The model under review builds one solid part; all positions refer to its coordinate system, in mm. A direction names the side the tool comes from. Coordinates: 2 decimals unless noted, no trailing zeros. Write each loop counter-clockwise with the first axis right and the second up, starting at its lowest first coordinate (ties: lowest second). Pieces come first, ordered by that corner, then holes. Notation, with made-up numbers: (34.25, 70.25) - (69.25, 70.25) arc R26 cw to (69.25, 90.25) - close; hole circle Ø5 at (-8.75, -38). An arc over 180 degrees is marked (long way). Put each result on its own line as item: value. Start each with the question number.
Item 1: Consider section C-C on z = 177.8. Give the boundary of the cut face in (x, y).
Item 2: Consider section B-B on x = 259. Give the boundary of the cut face in (y, z).
Item 3: Mouldability with a two-part tool opening along Z and no side actions: class faces 4 (the face through (-305, 188, -247.65)), 5 (the face through (5, 0, -4)), 6 (the face through (244, 127, 177)) as pulls with the +Z half, pulls with the -Z half, needs draft (parallel to the pull), parting line crosses it, or undercut.
Item 4: For pin 1 (5 mm diameter, centred on y = 232.5, z = -250, fed in from +X); pin 2 (15 mm diameter, centred on x = 11, y = 207, fed in from -Z), all flat-tipped, find the tip position at first contact; note any pin that passes through.
Item 5: To check wall thickness, follow L1, parallel to X at y = 75, z = -177; L2, parallel to X at y = 46.5, z = 177.8; L3, parallel to X at y = 342.5, z = -9. State the ranges of each line that lie inside material, in increasing order. Write a range as [from, to].
Item 6: Consider section D-D on x = 12.5. Give the boundary of the cut face in (y, z).
Item 7: Consider section A-A on z = 0. Give the boundary of the cut face in (x, y), then the cut area to 3 significant figures.
Item 8: Machinability: for faces 1 (the face through (0, 188, 247.65)), 2 (the face through (245, 127, -177)), 3 (the face through (5, 381, -4)), which of the approach directions +Z, -Z, +X, -X, +Y, -Y give a long, thin tool a straight path to every point of the face, cutting with its end or side? Answer none if there is none.
```python
from build123d import *

# Parameters (mm, degrees)
BOSS_EXTRUDE1_DEPTH = 381
BOSS_EXTRUDE2_DEPTH = 12.7
SKETCH4_R           = 21.592305898
CUT_EXTRUDE1_DEPTH  = 25.4
FILLET1_R           = 7.62
SKETCH5_R           = 25.4
CUT_EXTRUDE2_DEPTH  = 127


with BuildPart() as part:
    # Sketch2 → Boss-Extrude1 (new body)
    with BuildSketch(Plane(origin=(0, 0, 0), x_dir=(1, 0, 0), z_dir=(0, 1, 0))):
        Polygon((-381, 254), (-330.2, 254), (-330.2, 247.65), (-279.4, 247.65), (-279.4, 254), (-228.6, 254), (-228.6, 247.65), (-177.8, 247.65), (-177.8, 254), (-127, 254), (-127, 247.65), (-76.2, 247.65), (-76.2, 254), (-25.4, 254), (-25.4, 247.65), (25.4, 247.65), (25.4, 254), (76.2, 254), (76.2, 247.65), (127, 247.65), (127, 254), (177.8, 254), (177.8, 247.65), (228.6, 247.65), (228.6, 254), (279.4, 254), (279.4, 247.65), (330.2, 247.65), (330.2, 254), (381, 254), (381, -254), (330.2, -254), (330.2, -247.65), (279.4, -247.65), (279.4, -254), (228.6, -254), (228.6, -247.65), (177.8, -247.65), (177.8, -254), (127, -254), (127, -247.65), (76.2, -247.65), (76.2, -254), (25.4, -254), (25.4, -247.65), (-25.4, -247.65), (-25.4, -254), (-76.2, -254), (-76.2, -247.65), (-127, -247.65), (-127, -254), (-177.8, -254), (-177.8, -247.65), (-228.6, -247.65), (-228.6, -254), (-279.4, -254), (-279.4, -247.65), (-330.2, -247.65), (-330.2, -254), (-381, -254), align=None)
    extrude(amount=BOSS_EXTRUDE1_DEPTH)

    # Sketch3 → Boss-Extrude2 (add, symmetric)
    with BuildSketch(Plane(origin=(0, 68.58, 0), x_dir=(-1, 0, 0), z_dir=(0, -1, 0))):
        with BuildLine():
            Line((-458.892414986, -15.684101321), (-381, -69.382839719))
            Line((-381, -69.382839719), (-381, 69.382839719))
            Line((-381, 69.382839719), (-458.892414986, 15.684101321))
            ThreePointArc((-458.892414986, 15.684101321), (-467.12985443, 0), (-458.892414986, -15.684101321))
        make_face()
    extrude(amount=BOSS_EXTRUDE2_DEPTH, both=True)

    # Sketch4 → Cut-Extrude1 (cut)
    with BuildSketch(Plane(origin=(0, 81.28, 0), x_dir=(1, 0, 0), z_dir=(0, 1, 0))):
        with Locations(Location((429.496611066, 0, 0), (0, 0, 270))):
            Circle(SKETCH4_R)
    extrude(amount=-CUT_EXTRUDE1_DEPTH, mode=Mode.SUBTRACT)

    # Fillet1
    fillet1_edges = [part.edges().sort_by_distance(p)[0] for p in [
        (419.946207493, 81.28, -42.53347052),
        (467.12985443, 81.28, 0),
        (419.946207493, 81.28, 42.53347052),
        (419.946207493, 55.88, -42.53347052),
        (467.12985443, 55.88, 0),
        (419.946207493, 55.88, 42.53347052),
    ]]
    fillet(fillet1_edges, radius=FILLET1_R)

    # Sketch5 → Cut-Extrude2 (cut)
    with BuildSketch(Plane.XZ):
        with Locations(Location((-314.062017965, -177.8, 0), (0, 0, 270))):
            Circle(SKETCH5_R)
        with Locations(Location((244.737982035, -177.8, 0), (0, 0, 270))):
            Circle(SKETCH5_R)
        with Locations(Location((244.737982035, 177.8, 0), (0, 0, 90))):
            Circle(SKETCH5_R)
        with Locations(Location((-314.062017965, 177.8, 0), (0, 0, 90))):
            Circle(SKETCH5_R)
    extrude(amount=-CUT_EXTRUDE2_DEPTH, mode=Mode.SUBTRACT)


solid = part.part
```
Report:
1. outline: (-381, 0) - (-339.46, 0) - (-339.46, 127) - (-288.66, 127) - (-288.66, 0) - (219.34, 0) - (219.34, 127) - (270.14, 127) - (270.14, 0) - (381, 0) - (381, 381) - (-381, 381) - close
2. outline: (0, -254) - (381, -254) - (381, 254) - (0, 254) - (0, 198.82) - (127, 198.82) - (127, 156.78) - (0, 156.78) - (0, -156.78) - (127, -156.78) - (127, -198.82) - (0, -198.82) - close
3. face 4: pulls with the -Z half
3. face 5: needs draft
3. face 6: undercut
4. pin 1: x = 381
4. pin 2: z = -247.65
5. L1: [-381, -339.45], [-288.67, 219.35], [270.13, 381]
5. L2: [-381, -339.46], [-288.66, 219.34], [270.14, 381]
5. L3: [-381, 381]
6. outline: (0, -247.65) - (381, -247.65) - (381, 247.65) - (0, 247.65) - close
7. outline: (-381, 0) - (381, 0) - (381, 55.88) - (407.9, 55.88) - (407.9, 81.28) - (381, 81.28) - (381, 381) - (-381, 381) - close; (451.09, 55.88) - (459.51, 55.88) arc R7.62 ccw to (467.13, 63.5) - (467.13, 73.66) arc R7.62 ccw to (459.51, 81.28) - (451.09, 81.28) - close
7. area: 291,000 mm²
8. face 1: +Z, +Y, -Y
8. face 2: -Y
8. face 3: +Z, -Z, +X, -X, +Y
